Geometry check sheet. Reference: the model listing, model coordinates, mm. Coordinates: 2 decimals unless noted, no trailing zeros. Write each loop counter-clockwise with the first axis right and the second up, starting at its lowest first coordinate (ties: lowest second). Pieces come first, ordered by that corner, then holes. Notation, with made-up numbers: (45, -7) -> (90, -7) arc R7 cw to (90, 4) -> close; hole circle Ø8 at (89, 72). An arc over 180 degrees is marked (long way). Answer in a Markdown table with one row per item. Add a question column.
Q1. Thickness scan on line 1 (X direction, y = -2.4, z = 4.4); line 2 (X direction, y = -1.2, z = -5.5); line 3 (Z direction, x = -83.8, y = -1.5). Record the ranges inside material, lowest first.
Q2. Section check A-A, the plane y = -1. Record the boundary of the cut face in (x, z).
Q3. Section check D-D, the plane z = 3.75. Count the separate pieces of the cut face and the enclosed holes in it, and give its area (3 significant figures).
Q4. Section check B-B, the plane x = -83.8. Record the boundary of the cut face in (y, z) (3 decimals).
Q5. Section check C-C, the plane x = 0. Record the boundary of the cut face in (y, z) (3 decimals).
Q6. Gauge pin test, flat ends, axial feed: P1, Ø0.5, axis at x = 13, y = -2.5, coming from the +Z side; P2, Ø7.5, axis at x = 15, z = 0, coming from the +Y side; P3, Ø0.8, axis at x = 12.5, y = -2.5, coming from the -Z side. Record the tip position at first contact, or that the pin passes through.
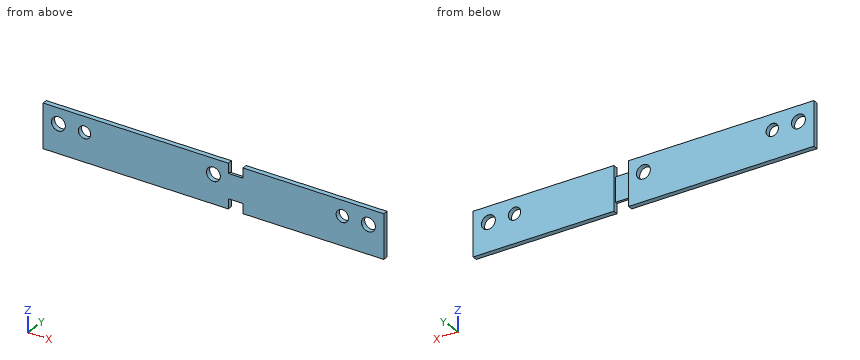
```python
from build123d import *

# Parameters (mm, degrees)
SKETCH1_W                      = 221.6
SKETCH1_H                      = 28.8
BOSS_EXTRUDE1_DEPTH            = 3.2
CUT_EXTRUDE1_REACH             = 113.778
SKETCH2_W                      = 9.5
SKETCH2_H                      = 6.4
CUT_EXTRUDE2_REACH             = 115.087
SKETCH3_W                      = 9.5
SKETCH3_H                      = 1.6
M8_CLEARANCE_HOLE1_AT_2_COUNT  = 2
M8_CLEARANCE_HOLE1_AT_2_PITCH  = 201.6
M8_CLEARANCE_HOLE1_AT_3_COUNT  = 2
M8_CLEARANCE_HOLE1_AT_3_PITCH  = 100.8
F_8_0MM_DOWEL_HOLE1_AT_2_COUNT = 2
F_8_0MM_DOWEL_HOLE1_AT_2_PITCH = 167.6


with BuildPart() as part:
    # Sketch1 → Boss-Extrude1 (new body)
    with BuildSketch(Plane(origin=(0, 0, 0), x_dir=(1, 0, 0), z_dir=(0, 1, 0))):
        Rectangle(SKETCH1_W, SKETCH1_H)
    extrude(amount=-BOSS_EXTRUDE1_DEPTH)

    # Sketch2 → Cut-Extrude1 (cut, up to next)
    with BuildSketch(Plane(origin=(0, 0, 0), x_dir=(1, 0, 0), z_dir=(0, 1, 0)), mode=Mode.PRIVATE) as cut_extrude1_sk1:
        with Locations((14.45, 11.2)):
            Rectangle(SKETCH2_W, SKETCH2_H)
    cut_extrude1_tool1 = extrude(cut_extrude1_sk1.sketch, amount=-CUT_EXTRUDE1_REACH, mode=Mode.PRIVATE) & part.part
    # Sketch2 → Cut-Extrude1 (cut, up to next)
    with BuildSketch(Plane(origin=(0, 0, 0), x_dir=(1, 0, 0), z_dir=(0, 1, 0)), mode=Mode.PRIVATE) as cut_extrude1_sk2:
        with Locations((14.45, -11.2)):
            Rectangle(SKETCH2_W, SKETCH2_H)
    cut_extrude1_tool2 = extrude(cut_extrude1_sk2.sketch, amount=-CUT_EXTRUDE1_REACH, mode=Mode.PRIVATE) & part.part
    add(cut_extrude1_tool1.solids().sort_by_distance((14.45, 0, -11.2))[0], mode=Mode.SUBTRACT)
    add(cut_extrude1_tool2.solids().sort_by_distance((14.45, 0, 11.2))[0], mode=Mode.SUBTRACT)

    # Sketch3 → Cut-Extrude2 (cut, up to next)
    with BuildSketch(Plane.XY.offset(8), mode=Mode.PRIVATE) as cut_extrude2_sk1:
        with Locations((14.45, -0.8)):
            Rectangle(SKETCH3_W, SKETCH3_H)
    cut_extrude2_tool1 = extrude(cut_extrude2_sk1.sketch, amount=-CUT_EXTRUDE2_REACH, mode=Mode.PRIVATE) & part.part
    add(cut_extrude2_tool1.solids().sort_by_distance((14.45, -0.8, 8))[0], mode=Mode.SUBTRACT)

    # Sketch5 → M8 Clearance Hole1 (revolve, cut)
    with BuildSketch(Plane(origin=(-100.8, 0, 4.4), x_dir=(0, 0, 1), z_dir=(1, 0, 0))):
        Polygon((0, 0), (0, 3.2), (4.525, 3.2), (4.5, 3.175), (4.5, 0.025), (4.525, 0), align=None)
    m8_clearance_hole1 = revolve(axis=Axis((-100.8, 6.35, 4.4), (0, -1, 0)), mode=Mode.SUBTRACT)

    # M8 Clearance Hole1 at 2: M8 Clearance Hole1 ×2
    with Locations(*[(i * M8_CLEARANCE_HOLE1_AT_2_PITCH, 0, 0) for i in range(1, M8_CLEARANCE_HOLE1_AT_2_COUNT)]):
        add(m8_clearance_hole1, mode=Mode.SUBTRACT)

    # M8 Clearance Hole1 at 3: M8 Clearance Hole1 ×2
    with Locations(*[(i * M8_CLEARANCE_HOLE1_AT_3_PITCH, 0, 0) for i in range(1, M8_CLEARANCE_HOLE1_AT_3_COUNT)]):
        add(m8_clearance_hole1, mode=Mode.SUBTRACT)

    # Sketch7 → Ø8.0mm Dowel Hole1 (revolve, cut)
    with BuildSketch(Plane(origin=(83.8, 0, 4.4), x_dir=(0, 0, 1), z_dir=(1, 0, 0))):
        Polygon((0, 0), (0, 3.2), (4.025, 3.2), (4, 3.175), (4, 0.025), (4.025, 0), align=None)
    f_8_0mm_dowel_hole1 = revolve(axis=Axis((83.8, 6.35, 4.4), (0, -1, 0)), mode=Mode.SUBTRACT)

    # Ø8.0mm Dowel Hole1 at 2: Ø8.0mm Dowel Hole1 ×2
    with Locations(*[(-i * F_8_0MM_DOWEL_HOLE1_AT_2_PITCH, 0, 0) for i in range(1, F_8_0MM_DOWEL_HOLE1_AT_2_COUNT)]):
        add(f_8_0mm_dowel_hole1, mode=Mode.SUBTRACT)


solid = part.part
```
Calculated:
| question | item | result |
|---|---|---|
| 1 | line 1 | x = -110.8 to -105.3, -96.3 to -87.8, -79.8 to -4.5, 4.5 to 79.8, 87.8 to 96.3, 105.3 to 110.8 |
| 1 | line 2 | x = -110.8 to 9.7, 19.2 to 110.8 |
| 1 | line 3 | z = -14.4 to 0.4, 8.4 to 14.4 |
| 2 | outline | (-110.8, -14.4) -> (9.7, -14.4) -> (9.7, 14.4) -> (-110.8, 14.4) -> close; (19.2, -14.4) -> (110.8, -14.4) -> (110.8, 14.4) -> (19.2, 14.4) -> close; hole circle Ø9 at (-100.8, 4.4); hole circle Ø8 at (-83.8, 4.4); hole circle Ø9 at (0, 4.4); hole circle Ø8 at (83.8, 4.4); hole circle Ø9 at (100.8, 4.4) |
| 3 | separate pieces | 6 |
| 3 | enclosed holes | 0 |
| 3 | area | 558 mm² |
| 4 | outline | (-3.2, -14.4) -> (0, -14.4) -> (0, 0.375) -> (-0.025, 0.4) -> (-3.175, 0.4) -> (-3.2, 0.375) -> close; (-3.2, 8.425) -> (-3.175, 8.4) -> (-0.025, 8.4) -> (0, 8.425) -> (0, 14.4) -> (-3.2, 14.4) -> close |
| 5 | outline | (-3.2, -14.4) -> (0, -14.4) -> (0, -0.125) -> (-0.025, -0.1) -> (-3.175, -0.1) -> (-3.2, -0.125) -> close; (-3.2, 8.925) -> (-3.175, 8.9) -> (-0.025, 8.9) -> (0, 8.925) -> (0, 14.4) -> (-3.2, 14.4) -> close |
| 6 | P1 | stops at z = 8 |
| 6 | P2 | stops at y = -1.6 |
| 6 | P3 | stops at z = -8 |
